from build123d import *

# Parameters (mm, degrees)
SKETCH_1_W          = 40
SKETCH_1_H          = 75
EXTRUDE_1_DEPTH     = 21
FILLET_1_R          = 20
CHAMFER_1_SIZE      = 10
EXTRUDE_2_DEPTH     = 700
SKETCH_3_R          = 19
EXTRUDE_4_DEPTH     = 74
SKETCH_4_W          = 17
SKETCH_4_H          = 17
EXTRUDE_5_DEPTH     = 19
SKETCH_5_R          = 3
CUT_EXTRUDE_1_DEPTH = 19
SKETCH_6_R          = 10
EXTRUDE_6_DEPTH     = 16.5
SKETCH_7_R          = 12.75
EXTRUDE_7_DEPTH     = 20
SKETCH_9_R          = 2.9
CUT_EXTRUDE_2_DEPTH = 741.578996462


with BuildPart() as part:
    # 草图1 → 凸台-拉伸1 (new body)
    with BuildSketch(Plane.XY):
        Rectangle(SKETCH_1_W, SKETCH_1_H)
    extrude(amount=EXTRUDE_1_DEPTH)

    # 圆角1
    fillet_1_edges = [part.edges().sort_by_distance(p)[0] for p in [
        (-20, 37.5, 10.5),
        (20, 37.5, 10.5),
    ]]
    fillet(fillet_1_edges, radius=FILLET_1_R - 0.0001)  # a hair under: the kernel refuses the full size

    # 倒角1
    chamfer_1_edges = [part.edges().sort_by_distance(p)[0] for p in [
        (20, -37.5, 10.5),
        (-20, -37.5, 10.5),
    ]]
    chamfer(chamfer_1_edges, length=CHAMFER_1_SIZE)

    # 草图2 → 凸台-拉伸2 (add)
    with BuildSketch(Plane(origin=(0, 0, 0), x_dir=(-1, 0, 0), z_dir=(0, 0, -1))):
        with BuildLine():
            Line((-10, -37.5), (10, -37.5))
            Line((10, -37.5), (14.449874371, -21.525062814))
            ThreePointArc((14.449874371, -21.525062814), (0, -2.5), (-14.449874371, -21.525062814))
            Line((-14.449874371, -21.525062814), (-10, -37.5))
        make_face()
    extrude(amount=EXTRUDE_2_DEPTH)

    # 草图3 → 凸台-拉伸4 (add)
    with BuildSketch(Plane(origin=(0, 0, 0), x_dir=(-1, 0, 0), z_dir=(0, 0, -1))):
        with Locations(Location((0, 17.5, 0), (0, 0, 180))):
            Circle(SKETCH_3_R)
    extrude(amount=EXTRUDE_4_DEPTH)

    # 草图4 → 凸台-拉伸5 (add)
    with BuildSketch(Plane.XY.offset(21)):
        with Locations((0, -16.5)):
            Rectangle(SKETCH_4_W, SKETCH_4_H)
    extrude(amount=EXTRUDE_5_DEPTH)

    # 草图5 → 切除-拉伸1 (cut)
    with BuildSketch(Plane.ZY.offset(8.5)):
        with Locations(Location((31.5, -16.5, 0), (0, 0, 270))):
            Circle(SKETCH_5_R)
    extrude(amount=-CUT_EXTRUDE_1_DEPTH, mode=Mode.SUBTRACT)

    # 草图6 → 凸台-拉伸6 (add)
    with BuildSketch(Plane(origin=(0, 0, -700), x_dir=(-1, 0, 0), z_dir=(0, 0, -1))):
        with Locations((0, -17.5)):
            Circle(SKETCH_6_R)
    extrude(amount=EXTRUDE_6_DEPTH)

    # 草图7 → 凸台-拉伸7 (add)
    with BuildSketch(Plane(origin=(0, 0, -716.5), x_dir=(-1, 0, 0), z_dir=(0, 0, -1))):
        with Locations((0, -17.5)):
            Circle(SKETCH_7_R)
    extrude(amount=EXTRUDE_7_DEPTH)

    # 草图9 → 切除-拉伸2 (cut, through all)
    with BuildSketch(Plane.XZ.offset(37.5)):
        with Locations((0, -725.5)):
            Circle(SKETCH_9_R)
    extrude(amount=-CUT_EXTRUDE_2_DEPTH, mode=Mode.SUBTRACT)


solid = part.part
Geometry: final body of the model. Coordinates: model frame, mm. A direction names the side the tool comes from. Give positions to 0.01 mm unless a question says otherwise; leave off trailing zeros. Write each loop counter-clockwise with the first axis right and the second up, starting at its lowest first coordinate (ties: lowest second). Pieces come first, ordered by that corner, then holes.
(1) Access query for faces 4 (the flat face through (12.256, -29.401, -345.1)), 5 (the cylindrical face through (10.214, 1.479, -36.482)), 6 (the cylindrical face through (1.302, -7.585, -708.134)). Directions: +Z, -Z, +X, -X, +Y, -Y. A direction counts if a zero-diameter tool reaches every point of the face in a straight line with its end or side. Return the directions, or none.
(2) First-contact query: P1, Ø10, axis at x = 14, y = 2.5, coming from the -Z side; P2, Ø18.5, axis at y = -18.5, z = 33, coming from the -X side; P3, Ø6, axis at x = 15.5, z = -143, coming from the +Y side. Flat tips, straight axial feed; report the tip coordinate or a pass-through.
(3) Mould query, pull axis Z, two halves, no side actions, for faces 1 (the flat face through (8, -24, -716.5)), 2 (the flat face through (-20, -5, 10)), 3 (the flat face through (0, 17, -74)). Classes: released by +Z, released by -Z, zero draft, split by the parting line, or undercut.
(4) Cut plane A-A, the plane z = -104. Return loops of the section in (x, y), then the cut area to 3 significant figures.
(5) Ray query, line 1 (Z direction, x = -2, y = -16.5); line 2 (Z direction, x = 0, y = -13); line 3 (Z direction, x = 3.25, y = -16.5). Return the intervals inside material, ascending.
Values follow:
1. face 4: -Z, +X, -Y
1. face 5: -Z
1. face 6: none
2. P1: stops at z = -74
2. P2: stops at x = -8.5
2. P3: stops at y = -9.21
3. face 1: undercut
3. face 2: zero draft
3. face 3: released by -Z
4. outline: (-14.45, -21.53) - (-10, -37.5) - (10, -37.5) - (14.45, -21.53) arc R15 ccw (long way) to start
4. area: 863 mm2
5. line 1: z = -736.5 to -727.6, -723.4 to 28.5, 34.5 to 40
5. line 2: z = -736.5 to -728.4, -722.6 to 40
5. line 3: z = -736.5 to 28.5, 34.5 to 40
